from build123d import *

# Parameters (mm, degrees)
SKETCH1_W           = 279.4
SKETCH1_H           = 158.75
BOSS_EXTRUDE1_DEPTH = 2.667
SKETCH2_W           = 41.148
SKETCH2_H           = 41.148
CUT_EXTRUDE1_DEPTH  = 47.752
SKETCH3_R           = 2.7686
CUT_EXTRUDE2_DEPTH  = 322.361222597


with BuildPart() as part:
    # Sketch1 → Boss-Extrude1 (new body)
    with BuildSketch(Plane.XY):
        with Locations((139.7, 79.375)):
            Rectangle(SKETCH1_W, SKETCH1_H)
    extrude(amount=BOSS_EXTRUDE1_DEPTH)

    # Sketch2 → Cut-Extrude1 (cut)
    with BuildSketch(Plane.XY):
        with Locations((60.198, 131.318)):
            Rectangle(SKETCH2_W, SKETCH2_H)
    extrude(amount=CUT_EXTRUDE1_DEPTH, mode=Mode.SUBTRACT)

    # Sketch3 → Cut-Extrude2 (cut, through all)
    with BuildSketch(Plane.XY):
        with Locations((6.35, 9.525)):
            Circle(SKETCH3_R)
        with Locations((6.35, 79.375)):
            Circle(SKETCH3_R)
        with Locations((6.35, 149.225)):
            Circle(SKETCH3_R)
        with Locations((273.05, 9.525)):
            Circle(SKETCH3_R)
        with Locations((273.05, 79.375)):
            Circle(SKETCH3_R)
        with Locations((273.05, 149.225)):
            Circle(SKETCH3_R)
    extrude(amount=CUT_EXTRUDE2_DEPTH, mode=Mode.SUBTRACT)


solid = part.part
Check sheet for the modelled part. Datum: model origin and axes. Units: mm. Coordinates: 2 decimals unless noted, no trailing zeros. Loops run counter-clockwise (first coordinate to the right, second up) from the corner with the lowest first, then second, coordinate; pieces in that order, holes last. Notation, with made-up numbers: (-11.75, 3.5) -> (45.25, 3.5) arc R27 cw to (45.25, 35.5) -> close; hole circle Ø2 at (79.5, 80). An arc over 180 degrees is marked (long way). Write item = value, one per line. Start each with the question number.
1. Section check C-C on x = 273.05. Record the cut outline in (y, z), then the cut area to 3 significant figures.
2. Material ranges on line 1 (Y direction, x = 273.05, z = 2); line 2 (X direction, y = 140, z = 2.2); line 3 (X direction, y = 77.5, z = 0.6), recorded low to high.
3. Section check D-D on z = 1.55. Record the cut outline in (x, y) (3 decimals), then the cut area to 3 significant figures.
4. Draft check along Y on faces 1 (the flat face through (138, 80, 0)), 2 (the cylindrical face through (274.54, 81.71, 1.31)). Enter one of: released by +Y, released by -Y, zero draft, split by the parting line, or undercut.
5. Section check B-B on y = 140. Record the cut outline in (x, z), then the cut area to 3 significant figures.
6. Section check A-A on x = 46. Record the cut outline in (y, z).
Responses:
q1.outline = (0, 0) -> (6.76, 0) -> (6.76, 2.67) -> (0, 2.67) -> close; (12.29, 0) -> (76.61, 0) -> (76.61, 2.67) -> (12.29, 2.67) -> close; (82.14, 0) -> (146.46, 0) -> (146.46, 2.67) -> (82.14, 2.67) -> close; (151.99, 0) -> (158.75, 0) -> (158.75, 2.67) -> (151.99, 2.67) -> close
q1.area = 379 mm2
q2.line_1 = 0 to 6.76, 12.29 to 76.61, 82.14 to 146.46, 151.99 to 158.75
q2.line_2 = 0 to 39.62, 80.77 to 279.4
q2.line_3 = 0 to 4.31, 8.39 to 271.01, 275.09 to 279.4
q3.outline = (0, 0) -> (279.4, 0) -> (279.4, 158.75) -> (0, 158.75) -> close; hole circle Ø5.537 at (6.35, 9.525); hole circle Ø5.537 at (6.35, 79.375); hole circle Ø5.537 at (6.35, 149.225); hole (39.624, 110.744) -> (80.772, 110.744) -> (80.772, 151.892) -> (39.624, 151.892) -> close; hole circle Ø5.537 at (273.05, 9.525); hole circle Ø5.537 at (273.05, 79.375); hole circle Ø5.537 at (273.05, 149.225)
q3.area = 42,500 mm2
q4.face_1 = zero draft
q4.face_2 = undercut
q5.outline = (0, 0) -> (39.62, 0) -> (39.62, 2.67) -> (0, 2.67) -> close; (80.77, 0) -> (279.4, 0) -> (279.4, 2.67) -> (80.77, 2.67) -> close
q5.area = 635 mm2
q6.outline = (0, 0) -> (110.74, 0) -> (110.74, 2.67) -> (0, 2.67) -> close; (151.89, 0) -> (158.75, 0) -> (158.75, 2.67) -> (151.89, 2.67) -> close
